Geometry check sheet. Reference: the model listing, model coordinates, mm. A direction names the side the tool comes from. Give positions to 0.01 mm unless a question says otherwise; leave off trailing zeros. Loops run counter-clockwise (first coordinate to the right, second up) from the corner with the lowest first, then second, coordinate; pieces in that order, holes last. Notation, with made-up numbers: (26.25, -31.5) -> (83.25, -31.5) arc R32 cw to (83.25, 0.5) -> close; hole circle Ø8 at (19, 46.25). An arc over 180 degrees is marked (long way). One line per question, with ' | ' between items.
Autodesk Inventor part; units mm, degrees
ref_plane "YZ Plane" through (0, 0, 0) normal (1, 0, 0) x (0, 1, 0)
ref_plane "XZ Plane" through (0, 0, 0) normal (0, 1, 0) x (-1, 0, 0)
ref_plane "XY Plane" through (0, 0, 0) normal (0, 0, 1) x (1, 0, 0)
sketch "Sketch1" plane through (0, 0, 0) normal (1, 0, 0) x (0, 1, 0)
  line L0 (-5, 6) -> (5, 6)
  line L1 (5, 6) -> (5, -6)
  line L2 (5, -6) -> (-5, -6)
  line L3 (-5, -6) -> (-5, 6)
  line L4 (-5, 6) -> (5, -6) construction
  line L5 (5, 6) -> (-5, -6) construction
  point P0 (0, 0)
  dimension "d0" = 10
  dimension "d1" = 12
extrude "Extrusion1" add sketch "Sketch1" along normal blind 26.29
sketch "Sketch2" plane through (26.29, 0, 0) normal (1, 0, 0) x (0, 0, -1)
  circle A0 centre (0, 0) radius 1.5
  dimension "d4" = 3
fillet "Fillet1" radius 2 5 edges at (13.145, 5, 6) (13.145, 5, -6) (13.145, -5, 6) (13.145, -5, -6) (0, 5, 0)
extrude "Extrusion2" add sketch "Sketch2" along normal blind 9.1
properties part number "motor" material "Aluminum 6061"
Item 1: Set-up check for faces 1 (the face through (13.33, 4.4, -5.43)), 2 (the face through (26.29, -1.2, -1.2)): record each of +Z, -Z, +X, -X, +Y, -Y from which the full face is reachable in a straight line by a thin tool's end or side.
Result:
face 1: -Z, +X, -X, +Y | face 2: +X
Item 2: Sectioned sample at B-B (x = 7). Record the cut outline in (y, z).
Result:
outline: (-5, -4) arc R2 ccw to (-3, -6) -> (3, -6) arc R2 ccw to (5, -4) -> (5, 4) arc R2 ccw to (3, 6) -> (-3, 6) arc R2 ccw to (-5, 4) -> close
Item 3: Sectioned sample at C-C (y = 0). Record the cut outline in (x, z).
Result:
outline: (0, -6) -> (26.29, -6) -> (26.29, -1.5) -> (35.39, -1.5) -> (35.39, 1.5) -> (26.29, 1.5) -> (26.29, 6) -> (0, 6) -> close
Item 4: Sectioned sample at D-D (z = -2.5). Record the cut outline in (x, y).
Result:
outline: (0, -5) -> (26.29, -5) -> (26.29, 5) -> (2, 5) arc R2 ccw to (0, 3) -> close
Item 5: Sectioned sample at A-A (z = 0). Record the cut outline in (x, y).
Result:
outline: (0, -5) -> (26.29, -5) -> (26.29, -1.5) -> (35.39, -1.5) -> (35.39, 1.5) -> (26.29, 1.5) -> (26.29, 5) -> (2, 5) arc R2 ccw to (0, 3) -> close
Item 6: Scan lines: probe 1 along X at (y, z) = (-2, -4.75); probe 2 along X at (y, z) = (4.75, -1); probe 3 along Z at (x, y) = (23, 3.25). Record each from-to range of solid material in increasing order.
Result:
probe 1: 0 to 26.29 | probe 2: 1.03 to 26.29 | probe 3: -5.98 to 5.98
